Could you check a few things on this drawing? It's one solid part, dimensions in mm from its lowest x, y, z. Coordinates: 2 decimals unless noted, no trailing zeros. Write each loop counter-clockwise with the first axis right and the second up, starting at its lowest first coordinate (ties: lowest second). Pieces come first, ordered by that corner, then holes. Notation, with made-up numbers: M 26,-15.5 L 36,-15.5 A33 cw 36,16.5 Z; hole C 31.25,30 d4. An arc over 180 degrees is marked long. Use a Markdown table: item, result.
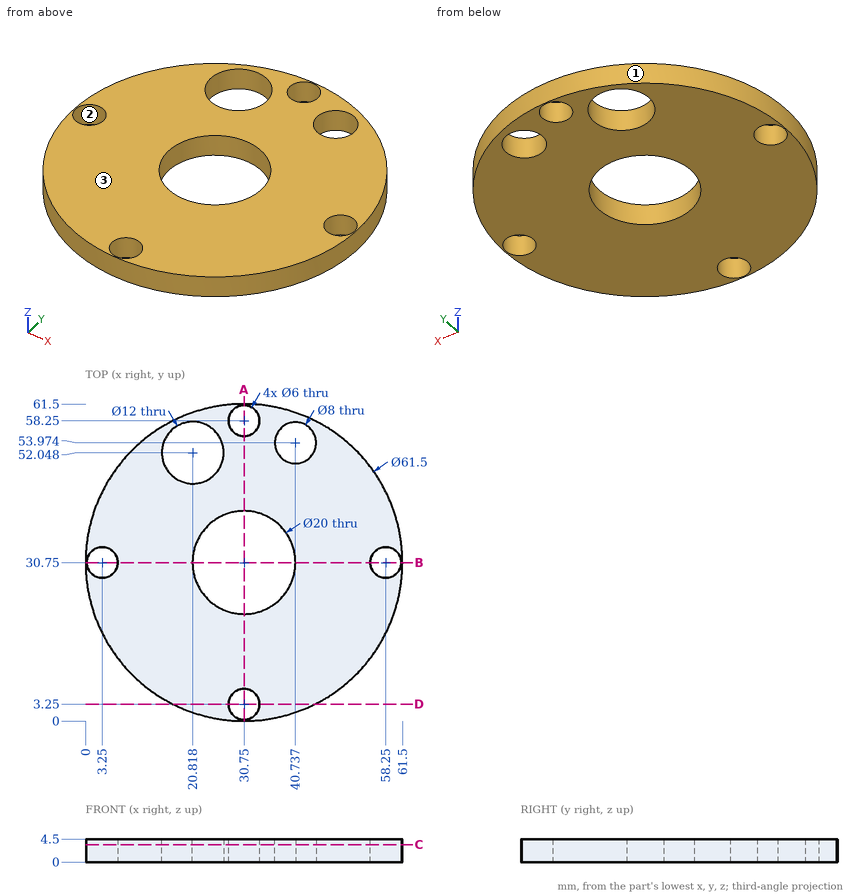
1. Suppose I cut it at A-A on x = 30.75. Write out the boundary of the cut face in (y, z), and give its area (3 significant figures).
Answers follow:
| item | result |
|---|---|
| outline | M 0,0 L 0.25,0 L 0.25,4.5 L 0,4.5 Z; M 6.25,0 L 20.75,0 L 20.75,4.5 L 6.25,4.5 Z; M 40.75,0 L 55.25,0 L 55.25,4.5 L 40.75,4.5 Z; M 61.25,0 L 61.5,0 L 61.5,4.5 L 61.25,4.5 Z |
| area | 133 mm2 |
2. I need wall thicknesses on probe 1 along Y at (x, z) = (30.75, 3.35); probe 2 along X at (y, z) = (33, 0.3) (1 decimal); probe 3 along Y at (x, z) = (34, 3.05). Which ranges of each line are inside material? Lowest first, please.
Answers follow:
| item | result |
|---|---|
| probe 1 | y = 0 to 0.25, 6.25 to 20.75, 40.75 to 55.25, 61.25 to 61.5 |
| probe 2 | x = 0.1 to 1.3, 5.2 to 21, 40.5 to 56.3, 60.2 to 61.4 |
| probe 3 | y = 0.17 to 21.29, 40.21 to 61.33 |
3. We'd pull the mould along Y, two halves only. Please class the marked faces 1, 2 and 3: +Y half, -Y half, draft (parallel to the pull), parting line (faces both ways), or undercut.
Answers follow:
| item | result |
|---|---|
| face 1 | parting line |
| face 2 | undercut |
| face 3 | draft |
4. Suppose I cut it at D-D on y = 3.25. Write out the boundary of the cut face in (x, z).
Answers follow:
| item | result |
|---|---|
| outline | M 16.99,0 L 27.75,0 L 27.75,4.5 L 16.99,4.5 Z; M 33.75,0 L 44.51,0 L 44.51,4.5 L 33.75,4.5 Z |
5. Will these pins go through, and if not, where does the flat tip stop? pin 1 Ø5.5 at (x, y) = (30.75, 3.25) entering from +Z; pin 2 Ø1 at (y, z) = (30, 2.5) entering from +X; pin 3 Ø1 at (y, z) = (54.5, 0.5) entering from +X (1 decimal).
Answers follow:
| item | result |
|---|---|
| pin 1 | passes through |
| pin 2 | stops at x = 61.5 |
| pin 3 | stops at x = 50.9 |
6. Suppose I cut it at C-C on z = 3.4. State how many separate pieces and enclosed holes the cut face has, and give its area (3 significant figures).
Answers follow:
| item | result |
|---|---|
| separate pieces | 1 |
| enclosed holes | 7 |
| area | 2,380 mm2 |
